Geometry check sheet. Reference: the model listing, model coordinates, mm. Face numbers are marked on the shaded views. A direction names the side the tool comes from. Round coordinates to 2 decimals unless told otherwise and drop trailing zeros. Write each loop counter-clockwise with the first axis right and the second up, starting at its lowest first coordinate (ties: lowest second). Pieces come first, ordered by that corner, then holes. Notation, with made-up numbers: M -20.75,45 L 18.25,45 A36 cw 18.25,80 Z; hole C 28.25,69.5 d8. An arc over 180 degrees is marked long. Put each result on its own line as item: value. Start each with the question number.
(1) Tool access check on the marked faces 1, 2, 3 and 4. Record the directions out of +Z, -Z, +X, -X, +Y, -Y that give a thin tool (end or side, any length) a straight path to the whole face; none if there is none.
(2) Section check B-B on x = 16. Record the cut outline in (y, z).
(3) Section check D-D on z = 1.75. Record the cut outline in (x, y).
(4) Gauge pin test, flat ends, axial feed: pin 1 (3 mm diameter, centred on x = -9, z = -1, fed in from +Y); pin 2 (3 mm diameter, centred on x = -7.21, z = -3.39, fed in from -Y); pin 3 (10 mm diameter, centred on x = 8.5, z = 1, fed in from -Y). Record the tip position at first contact, or that the pin passes through.
(5) Material ranges on probe 1 along X at (y, z) = (2, 3.75); probe 2 along Z at (x, y) = (19, 4.5); probe 3 along Z at (x, y) = (16.5, 1.25), recorded low to high.
(6) Section check C-C on z = -2.5. Record the cut outline in (x, y), then the cut area to 3 significant figures.
(7) Section check A-A on y = 1.5. Record the cut outline in (x, z), then the cut area to 3 significant figures.
from build123d import *

# Parameters (mm, degrees)
SKETCH1_W           = 35
SKETCH1_H           = 25
BOSS_EXTRUDE1_DEPTH = 6
SKETCH2_R           = 2.5
CUT_EXTRUDE1_DEPTH  = 6
SKETCH3_W           = 7.5
SKETCH3_H           = 25
REVOLVE1_ANGLE      = 180
CUT_EXTRUDE2_DEPTH  = 36


with BuildPart() as part:
    # Sketch1 → Boss-Extrude1 (new body)
    with BuildSketch(Plane(origin=(0, 0, 0), x_dir=(1, 0, 0), z_dir=(0, 1, 0))):
        with Locations((5.286458333, -4.114583333)):
            Rectangle(SKETCH1_W, SKETCH1_H)
    extrude(amount=BOSS_EXTRUDE1_DEPTH)

    # Sketch2 → Cut-Extrude1 (cut)
    with BuildSketch(Plane(origin=(0, 6, 0), x_dir=(1, 0, 0), z_dir=(0, 1, 0))):
        with Locations((-7.213541667, -11.614583333)):
            Circle(SKETCH2_R)
        with Locations((17.786458333, 3.385416667)):
            Circle(SKETCH2_R)
        with Locations((17.786458333, -11.614583333)):
            Circle(SKETCH2_R)
        with Locations((-7.213541667, 3.385416667)):
            Circle(SKETCH2_R)
    extrude(amount=-CUT_EXTRUDE1_DEPTH, mode=Mode.SUBTRACT)

    # Sketch3 → Revolve1 (revolve)
    with BuildSketch(Plane(origin=(0, 6, 0), x_dir=(1, 0, 0), z_dir=(0, 1, 0))):
        with Locations((9.036458333, -4.114583333)):
            Rectangle(SKETCH3_W, SKETCH3_H)
    revolve(axis=Axis((5.286458333, 6, -8.385416667), (0, 0, 1)), revolution_arc=REVOLVE1_ANGLE)

    # Sketch4 → Cut-Extrude2 (cut)
    with BuildSketch(Plane.XY.offset(16.614583333)):
        with BuildLine():
            ThreePointArc((9.286458333, 6), (5.286458333, 10), (1.286458333, 6))
            Line((1.286458333, 6), (9.286458333, 6))
        make_face()
        with BuildLine():
            Line((9.286458333, 6), (1.286458333, 6))
            ThreePointArc((1.286458333, 6), (5.286458333, 2), (9.286458333, 6))
        make_face()
        with BuildLine():
            ThreePointArc((9.286458333, 6), (5.286458333, 2), (1.286458333, 6))
            Line((1.286458333, 6), (1.286458333, 0))
            Line((1.286458333, 0), (9.286458333, 0))
            Line((9.286458333, 0), (9.286458333, 6))
        make_face()
    extrude(amount=-CUT_EXTRUDE2_DEPTH, mode=Mode.SUBTRACT)


solid = part.part
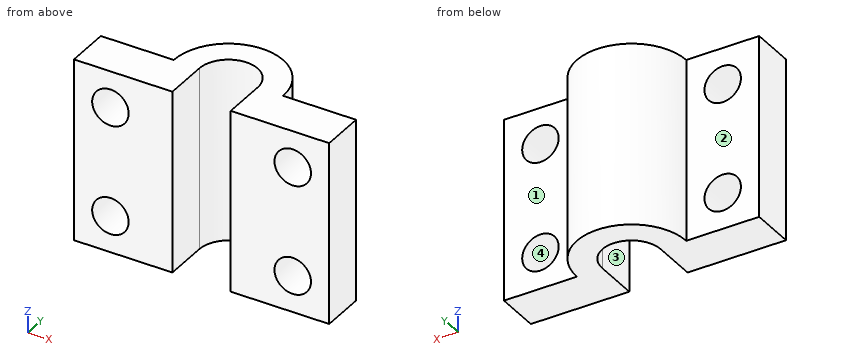
Answers follow:
1. face 1: +Z, -Z, +X, +Y
1. face 2: +Z, -Z, -X, +Y
1. face 3: +Z, -Z, -Y
1. face 4: +Y, -Y
2. outline: M 0,-8.39 L 6,-8.39 L 6,-5.13 L 0,-5.13 Z; M 0,-1.64 L 6,-1.64 L 6,9.87 L 0,9.87 Z; M 0,13.36 L 6,13.36 L 6,16.61 L 0,16.61 Z
3. outline: M -12.21,0 L 1.29,0 L 1.29,6 A4 cw 9.29,6 L 9.29,0 L 22.79,0 L 22.79,6 L 12.79,6 A7.5 ccw -2.21,6 L -12.21,6 Z
4. pin 1: stops at y = 6
4. pin 2: passes through
4. pin 3: stops at y = 0
5. probe 1: x = -12.21 to 1.29, 9.29 to 22.79
5. probe 2: z = -8.39 to -5.57, -1.2 to 9.43, 13.8 to 16.61
5. probe 3: z = -8.39 to -5.53, -1.24 to 9.47, 13.76 to 16.61
6. outline: M -12.21,0 L -9.55,0 L -9.55,6 L -12.21,6 Z; M -4.88,0 L 1.29,0 L 1.29,6 A4 cw 9.29,6 L 9.29,0 L 15.45,0 L 15.45,6 L 12.79,6 A7.5 ccw -2.21,6 L -4.88,6 Z; M 20.12,0 L 22.79,0 L 22.79,6 L 20.12,6 Z
6. area: 169 mm^2
7. outline: M -12.21,-8.39 L 1.29,-8.39 L 1.29,16.61 L -12.21,16.61 Z; M 9.29,-8.39 L 22.79,-8.39 L 22.79,16.61 L 9.29,16.61 Z; hole C -7.21,-3.39 d5; hole C -7.21,11.61 d5; hole C 17.79,-3.39 d5; hole C 17.79,11.61 d5
7. area: 596 mm^2
